Job drawing, mm, ordinate dimensions from the low corner. One solid piece. A direction names the side the tool comes from. Give positions to 0.01 mm unless a question says otherwise; leave off trailing zeros. Write each loop counter-clockwise with the first axis right and the second up, starting at its lowest first coordinate (ties: lowest second). Pieces come first, ordered by that corner, then holes. Notation, with made-up numbers: (-14, 30.25) -> (12, 30.25) arc R29 cw to (12, 50.25) -> close; hole circle Ø10 at (45.25, -7.75). An arc over 180 degrees is marked (long way). Put each result on its own line as item: value. Start each with the question number.
Item 1: Tool access for the marked faces 1 and 2: list every direction of +Z, -Z, +X, -X, +Y, -Y with a clear straight run to the whole face (end or side of a thin tool).
Item 2: Slice it at D-D, the plane y = 3.75. List the corners of the cut face in (x, z).
Item 3: Slice it at A-A, the plane x = 6.5. List the corners of the cut face in (y, z), plus the area to 3 significant figures.
Item 4: Slice it at C-C, the plane y = 1.5. List the corners of the cut face in (x, z).
Item 5: Drill centre lines: line 1 along Z through (x, y) = (6.5, 1.55); line 2 along Z through (x, y) = (4, 3.1); line 3 along X through (y, z) = (2.75, 6.5). Where is each one in solid material? Low to high.
Item 6: Slice it at B-B, the plane z = 6.5. List the corners of the cut face in (x, y).
Item 7: Flat gauge pins, fed straight in: pin 1 Ø1.5 at (y, z) = (1, 4) entering from +X; pin 2 Ø1.5 at (y, z) = (1, 1.5) entering from +X. Where does each tip first touch, or does it go through?
Item 8: Two-plate mould, pull along Z, no slides. Class the marked faces 3, 4 and 5: pulls with the +Z half, pulls with the -Z half, needs draft (parallel to the pull), parting line crosses it, or undercut.
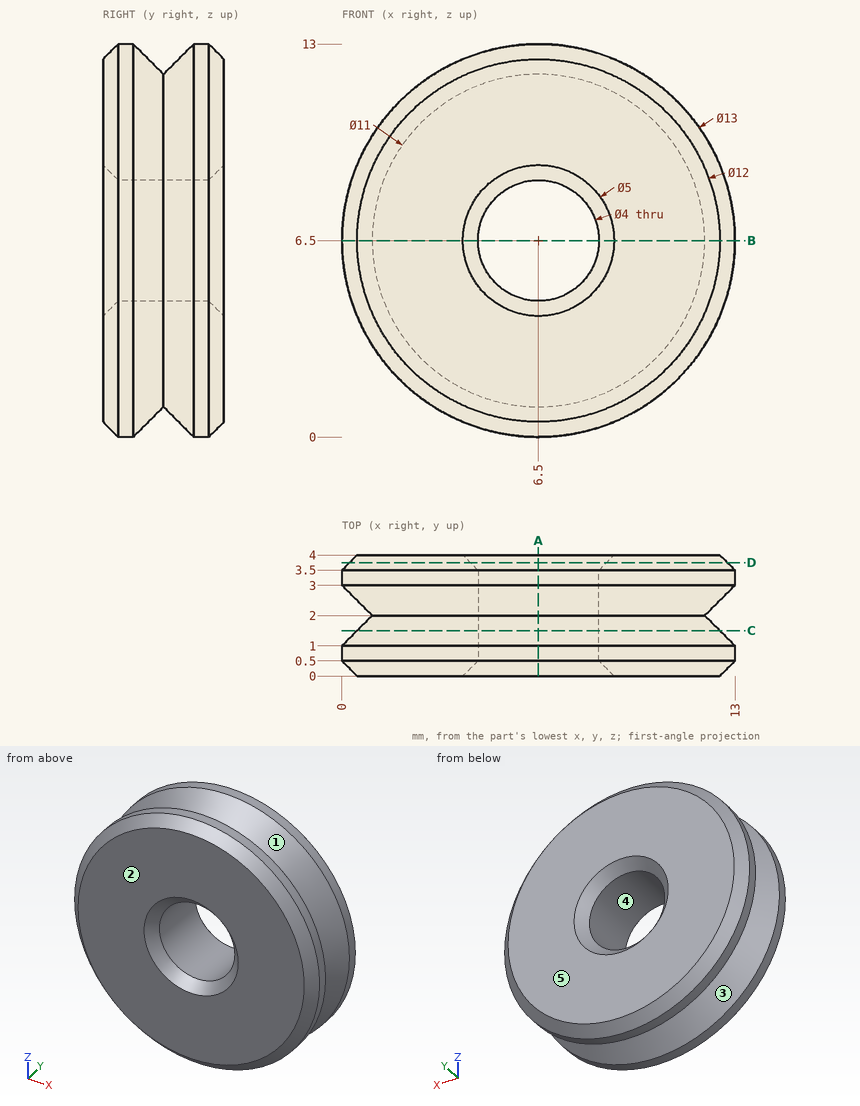
Values follow:
1. face 1: none
1. face 2: +Z, -Z, +X, -X, -Y
2. outline: circle Ø12.5 at (6.5, 6.5); hole circle Ø4.5 at (6.5, 6.5)
3. outline: (0, 0.5) -> (0.5, 0) -> (1, 0) -> (2, 1) -> (3, 0) -> (3.5, 0) -> (4, 0.5) -> (4, 4) -> (3.5, 4.5) -> (0.5, 4.5) -> (0, 4) -> close; (0, 9) -> (0.5, 8.5) -> (3.5, 8.5) -> (4, 9) -> (4, 12.5) -> (3.5, 13) -> (3, 13) -> (2, 12) -> (1, 13) -> (0.5, 13) -> (0, 12.5) -> close
3. area: 33.0 mm2
4. outline: circle Ø12 at (6.5, 6.5); hole circle Ø4 at (6.5, 6.5)
5. line 1: 0.55 to 4.5, 8.5 to 12.45
5. line 2: 0.5 to 12.5
5. line 3: 0.25 to 4.5, 8.5 to 12.75
6. outline: (0, 0.5) -> (0.5, 0) -> (4, 0) -> (4.5, 0.5) -> (4.5, 3.5) -> (4, 4) -> (0.5, 4) -> (0, 3.5) -> (0, 3) -> (1, 2) -> (0, 1) -> close; (8.5, 0.5) -> (9, 0) -> (12.5, 0) -> (13, 0.5) -> (13, 1) -> (12, 2) -> (13, 3) -> (13, 3.5) -> (12.5, 4) -> (9, 4) -> (8.5, 3.5) -> close
7. pin 1: x = 12.76
7. pin 2: x = 11.42
8. face 3: parting line crosses it
8. face 4: undercut
8. face 5: needs draft
